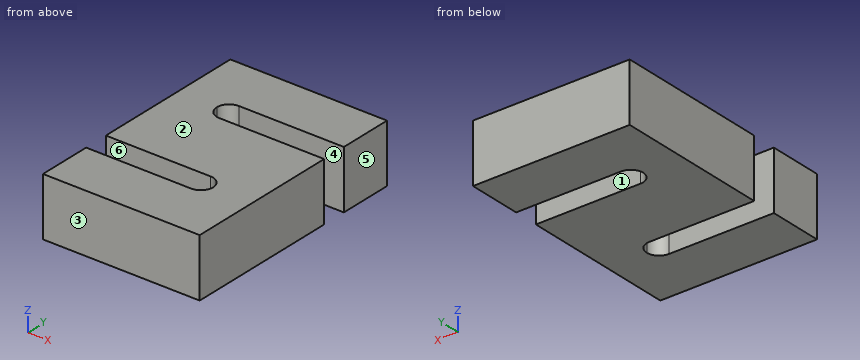
```python
from build123d import *

# Parameters (mm, degrees)
F0_W     = 50.8
F0_H     = 76
F1_DEPTH = 19
F3_DEPTH = 19.001
F5_DEPTH = 19.001


with BuildPart() as f1:
    # F0 (on Top) → F1 (new body)
    with BuildSketch(Plane.XY):
        Rectangle(F0_W, F0_H)
    extrude(amount=F1_DEPTH)

    # F2 (on face) → F3 (cut, through all)
    with BuildSketch(Plane.XY.offset(19)):
        with BuildLine():
            Line((-25.4, -12.5), (-25.4, -20.5))
            Line((-25.4, -20.5), (8.6, -20.5))
            ThreePointArc((8.6, -20.5), (11.428427, -19.328427), (12.6, -16.5))
            ThreePointArc((12.6, -16.5), (11.428427, -13.671573), (8.6, -12.5))
            Line((8.6, -12.5), (-25.4, -12.5))
        make_face()
    extrude(amount=-F3_DEPTH, mode=Mode.SUBTRACT)

    # F4 (on face) → F5 (cut, through all)
    with BuildSketch(Plane.XY.offset(19)):
        with BuildLine():
            Line((25.4, 12.5), (25.4, 20.5))
            Line((25.4, 20.5), (-8.6, 20.5))
            ThreePointArc((-8.6, 20.5), (-11.428427, 19.328427), (-12.6, 16.5))
            ThreePointArc((-12.6, 16.5), (-11.428427, 13.671573), (-8.6, 12.5))
            Line((-8.6, 12.5), (25.4, 12.5))
        make_face()
    extrude(amount=-F5_DEPTH, mode=Mode.SUBTRACT)


solid = f1.part
```
Geometry: final body of the model. Coordinates: model frame, mm. Face numbers are marked on the shaded views. A direction names the side the tool comes from. Coordinates: 2 decimals unless noted, no trailing zeros. Order: outer loops, then holes, each group sorted by start corner. A loop starts at its lowest first (then second) coordinate and runs counter-clockwise, first axis right, second up. Notation, with made-up numbers: (73.5, 62) - (80.5, 62) arc R34 cw to (80.5, 93) - close; hole circle Ø4 at (67.25, 79.5). An arc over 180 degrees is marked (long way). Write each question's results on one line, items separated by ' | '.
(1) First-contact query: pin 1 Ø1.5 at (x, y) = (9, 19) entering from +Z. Flat tip, straight axial feed; report the tip coordinate or a pass-through.
Values found:
pin 1: passes through
(2) Set-up query: the marked faces 5 and 6. Return all of +Z, -Z, +X, -X, +Y, -Y with unobstructed straight access to the full face (end or side cutting, diameter ignored); none if empty.
Values found:
face 5: +Z, -Z, +X, +Y, -Y | face 6: +Z, -Z, -X
(3) Section query D-D, the plane y = 14. Return the cut outline in (x, z), plus the area to 3 significant figures.
Values found:
outline: (-25.4, 0) - (-11.72, 0) - (-11.72, 19) - (-25.4, 19) - close | area: 260 mm²
(4) Line query: line 1 (Y direction, x = 3.5, z = 16.25); line 2 (Y direction, x = -19, z = 8.5); line 3 (Y direction, x = 13.5, z = 10.75). Output: solid intervals per line, ascending. Write a range as [from, to].
Values found:
line 1: y = [-38, -20.5], [-12.5, 12.5], [20.5, 38] | line 2: y = [-38, -20.5], [-12.5, 38] | line 3: y = [-38, 12.5], [20.5, 38]
(5) Section query A-A, the plane x = -2.5. Return the cut outline in (y, z), plus the area to 3 significant figures.
Values found:
outline: (-38, 0) - (-20.5, 0) - (-20.5, 19) - (-38, 19) - close; (-12.5, 0) - (12.5, 0) - (12.5, 19) - (-12.5, 19) - close; (20.5, 0) - (38, 0) - (38, 19) - (20.5, 19) - close | area: 1,140 mm²
(6) Section query B-B, the plane x = -18.5. Return the cut outline in (y, z).
Values found:
outline: (-38, 0) - (-20.5, 0) - (-20.5, 19) - (-38, 19) - close; (-12.5, 0) - (38, 0) - (38, 19) - (-12.5, 19) - close
(7) Section query C-C, the plane z = 12.25. Return the cut outline in (x, y).
Values found:
outline: (-25.4, -38) - (25.4, -38) - (25.4, 12.5) - (-8.6, 12.5) arc R4 cw to (-8.6, 20.5) - (25.4, 20.5) - (25.4, 38) - (-25.4, 38) - (-25.4, -12.5) - (8.6, -12.5) arc R4 cw to (8.6, -20.5) - (-25.4, -20.5) - close
(8) Mould query, pull axis Y, two halves, no side actions, for the marked faces 1, 2, 3 and 4. Classes: +Y half, -Y half, draft (parallel to the pull), parting line (faces both ways), or undercut.
Values found:
face 1: undercut | face 2: draft | face 3: -Y half | face 4: undercut
